Can you work these out from the model? Positions are in its coordinate system, mm. Round coordinates to 2 decimals unless told otherwise and drop trailing zeros. Loops run counter-clockwise (first coordinate to the right, second up) from the corner with the lowest first, then second, coordinate; pieces in that order, holes last.
(1) Will this pin go through, and if not, where does the flat tip stop? pin 1 Ø3 at (x, y) = (0, 69.5) entering from -Z.
(2) Thinking about a two-plate mould opening in X: for faces 1 (the face through (-0.234, 55.285, 2.888)), 2 (the face through (-29, 61, 3)), 3 (the face through (0, 62, -5)), which applies, released by +X, released by -X, zero draft, split by the parting line, or undercut?
(3) If I drill on line 1 along Y through (x, z) = (0, 1.25); line 2 along X through (y, z) = (69.5, 4.5); line 3 along X through (y, z) = (70, 8), over which ranges is the centre line in solid material (lowest first)?
(4) I want a section at B-B on y = 53.5. Write out the boundary of the cut face in (x, z), plus the area to 3 significant figures.
(5) I want a section at A-A on x = 0. Write out the boundary of the cut face in (y, z), plus the area to 3 significant figures.
from build123d import *

# Parameters (mm, degrees)
CYLINDER003_R     = 1.8
CYLINDER003_DEPTH = 50
ARRAY001_Y_COUNT  = 2
ARRAY001_Y_PITCH  = 16
BOX_W             = 58
BOX_H             = 32
BOX_DEPTH         = 16


with BuildPart() as bolt_hole_array:
    # Cylinder003 → Cylinder003 (new body)
    with BuildSketch(Plane.XY):
        Circle(CYLINDER003_R)
    extrude(amount=CYLINDER003_DEPTH)

    # Array001 Y: bolt hole array ×2


with BuildPart() as bolt_hole_array_1:
    add(bolt_hole_array.part)
    with Locations(*[(0, i * ARRAY001_Y_PITCH, 0) for i in range(1, ARRAY001_Y_COUNT)]):
        add(bolt_hole_array.part)


with BuildPart() as bolt_hole_array_2:
    # Array001 placement: moved
    add(bolt_hole_array_1.part.moved(Location((29, 8, 0))))


with BuildPart() as battery_mockup_cut:
    # Box → Box (new body)
    with BuildSketch(Plane.XY):
        with Locations((29, 16)):
            Rectangle(BOX_W, BOX_H)
    extrude(amount=BOX_DEPTH)

    # Cut002: cut bolt hole array
    add(bolt_hole_array_2.part, mode=Mode.SUBTRACT)


with BuildPart() as battery_mockup_cut_1:
    # Cut002 placement: moved
    add(battery_mockup_cut.part.moved(Location((-29, 45.5, -5))))


solid = battery_mockup_cut_1.part
Filled sheet:
1. pin 1: passes through
2. face 1: undercut
2. face 2: released by -X
2. face 3: zero draft
3. line 1: y = 45.5 to 51.7, 55.3 to 67.7, 71.3 to 77.5
3. line 2: x = -29 to -1.8, 1.8 to 29
3. line 3: x = -29 to -1.73, 1.73 to 29
4. outline: (-29, -5) - (-1.8, -5) - (-1.8, 11) - (-29, 11) - close; (1.8, -5) - (29, -5) - (29, 11) - (1.8, 11) - close
4. area: 870 mm2
5. outline: (45.5, -5) - (51.7, -5) - (51.7, 11) - (45.5, 11) - close; (55.3, -5) - (67.7, -5) - (67.7, 11) - (55.3, 11) - close; (71.3, -5) - (77.5, -5) - (77.5, 11) - (71.3, 11) - close
5. area: 397 mm2
